Source: CAD feature listing. Evaluate the final solid. Frame: model axes, mm. A direction names the side the tool comes from. Round coordinates to 2 decimals unless told otherwise and drop trailing zeros. Write each loop counter-clockwise with the first axis right and the second up, starting at its lowest first coordinate (ties: lowest second). Pieces come first, ordered by that corner, then holes. Notation, with made-up numbers: M 52.5,52.5 L 85.5,52.5 A32 ccw 85.5,84.5 Z; hole C -5.75,7.25 d7. An arc over 180 degrees is marked long. Use a Markdown table: item, result.
```python
from build123d import *


with BuildPart() as part:
    # Croquis1 → Revolución1 (revolve)
    with BuildSketch(Plane.XY, mode=Mode.PRIVATE) as revoluci_n1_sk:
        with BuildLine():
            Line((24, 7.15), (24, 6.5))
            Line((24, 6.5), (23, 6.5))
            Line((23, 6.5), (23, 7.1))
            Line((23, 7.1), (22, 7.1))
            Line((22, 7.1), (22, 5.5))
            Line((22, 5.5), (2, 5.5))
            Line((2, 5.5), (2, 6.8))
            Line((2, 6.8), (1, 6.8))
            Line((1, 6.8), (1, 6.5))
            Line((1, 6.5), (0, 6.5))
            Line((0, 6.5), (0, 7.15))
            ThreePointArc((0, 7.15), (0.102512627, 7.397487373), (0.35, 7.5))
            Line((0.35, 7.5), (3.25, 7.5))
            Line((3.25, 7.5), (3.25, 7.15))
            Line((3.25, 7.15), (4.35, 7.15))
            Line((4.35, 7.15), (4.35, 7.5))
            Line((4.35, 7.5), (19.65, 7.5))
            Line((19.65, 7.5), (19.65, 7.15))
            Line((19.65, 7.15), (20.75, 7.15))
            Line((20.75, 7.15), (20.75, 7.5))
            Line((20.75, 7.5), (23.65, 7.5))
            ThreePointArc((23.65, 7.5), (23.897487373, 7.397487373), (24, 7.15))
        make_face()
    revolve(revoluci_n1_sk.sketch.rotate(Axis((0, 0, 0), (1, 0, 0)), 90), axis=Axis((0, 0, 0), (1, 0, 0)))


solid = part.part
```
Q1. First-contact query: pin 1 Ø1.5 at (x, y) = (3.5, 4.5) entering from +Z; pin 2 Ø1.5 at (x, z) = (11.5, -3.5) entering from -Y; pin 3 Ø3 at (y, z) = (5.5, -5) entering from -X; pin 4 Ø7 at (y, z) = (0.5, -2.5) entering from +X. Flat tips, straight axial feed; report the tip coordinate or a pass-through.
Results are:
| item | result |
|---|---|
| pin 1 | z = 6.47 |
| pin 2 | y = -6.98 |
| pin 3 | x = 0 |
| pin 4 | x = 22 |
Q2. Reachability of faces 4 (the cylindrical face through (23.493, 3.955, -5.158)), 5 (the cylindrical face through (11.86, 5.37, -1.19)), 6 (the cylindrical face through (0.493, 3.955, -5.158)), 7 (the cylindrical face through (22.49, -7.04, -0.92)) from +Z, -Z, +X, -X, +Y, -Y: full face, straight path, thin tool, end or side. Return the list, or none.
Results are:
| item | result |
|---|---|
| face 4 | +X |
| face 5 | +X, -X |
| face 6 | -X |
| face 7 | none |
Q3. Section A-A on x = 14.75. Return loops of the section in (y, z), plus the area to 3 significant figures.
Results are:
| item | result |
|---|---|
| outline | C 0,0 d15; hole C 0,0 d11 |
| area | 81.7 mm^2 |
Q4. Line query: L1, parallel to Y at x = 10.5, z = 0; L2, parallel to Y at x = 23.35, z = 0; L3, parallel to X at y = -5, z = 5.25. Output: solid intervals per line, ascending.
Results are:
| item | result |
|---|---|
| L1 | -7.5 to -5.5, 5.5 to 7.5 |
| L2 | -7.5 to -6.5, 6.5 to 7.5 |
| L3 | 0.01 to 3.25, 4.35 to 19.65, 20.75 to 23.99 |
Q5. Mould query, pull axis Y, two halves, no side actions, for faces 1 (the cylindrical face through (3.81, -7.09, -0.93)), 2 (the flat face through (24, 6, 3)), 3 (the flat face through (23, 6, -3)). Classes: +Y half, -Y half, draft (parallel to the pull), parting line (faces both ways), or undercut.
Results are:
| item | result |
|---|---|
| face 1 | parting line |
| face 2 | draft |
| face 3 | undercut |
